The listing builds one solid part. Answer for the finished solid, in the listing's coordinates (mm). A direction names the side the tool comes from. Coordinates: 2 decimals unless noted, no trailing zeros. Write each loop counter-clockwise with the first axis right and the second up, starting at its lowest first coordinate (ties: lowest second). Pieces come first, ordered by that corner, then holes. Notation, with made-up numbers: M 10.25,3 L 30.25,3 A24 ccw 30.25,35 Z; hole C -1,58.5 d11. An arc over 180 degrees is marked long. Put each result on its own line as item: value. Start each with the question number.
```python
from build123d import *

# Parameters (mm, degrees)
SKETCH_1_R               = 2.5
EXTRUDE_1_DEPTH          = 86
HOLE_WIZARD_M3_1_D       = 2.5
HOLE_WIZARD_M3_1_DEPTH   = 6.748924226
HOLE_WIZARD_M3_1_TIP     = 0.751075774
HOLE_WIZARD_M3_2_D       = 2.5
HOLE_WIZARD_M3_2_DEPTH   = 6.748924226
HOLE_WIZARD_M3_2_TIP     = 0.751075774
CUT_EXTRUDE_2_DEPTH      = 5
CUT_EXTRUDE_2_DEPTH_BACK = 5
SKETCH_10_R              = 1.5
SKETCH_10_R_2            = 1.4


with BuildPart() as part:
    # Sketch 1 → Extrude 1 (new body)
    with BuildSketch(Plane(origin=(0, 0, 0), x_dir=(1, 0, 0), z_dir=(0, 1, 0))):
        with Locations(Location((0, 0, 0), (0, 0, 270))):
            Circle(SKETCH_1_R)
    extrude(amount=EXTRUDE_1_DEPTH)

    # Hole Wizard M3 _1
    with Locations(Plane(origin=(0, 0, 0), x_dir=(-1, 0, 0), z_dir=(0, -1, 0))):
        with Locations((0, 0)):
            Hole(HOLE_WIZARD_M3_1_D / 2, depth=HOLE_WIZARD_M3_1_DEPTH)
            with Locations((0, 0, -(HOLE_WIZARD_M3_1_DEPTH + HOLE_WIZARD_M3_1_TIP / 2))):  # 118° drill point
                Cone(0, HOLE_WIZARD_M3_1_D / 2, HOLE_WIZARD_M3_1_TIP, mode=Mode.SUBTRACT)

    # Hole Wizard M3 _2
    with Locations(Plane(origin=(0, 86, 0), x_dir=(1, 0, 0), z_dir=(0, 1, 0))):
        with Locations((0, 0)):
            Hole(HOLE_WIZARD_M3_2_D / 2, depth=HOLE_WIZARD_M3_2_DEPTH)
            with Locations((0, 0, -(HOLE_WIZARD_M3_2_DEPTH + HOLE_WIZARD_M3_2_TIP / 2))):  # 118° drill point
                Cone(0, HOLE_WIZARD_M3_2_D / 2, HOLE_WIZARD_M3_2_TIP, mode=Mode.SUBTRACT)

    # Sketch 10 → Cut-Extrude 2 (cut, two sides: drawn at the far end of the back side and taken through both)
    with BuildSketch(Plane(origin=(0, 0, 0), x_dir=(0, 0, -1), z_dir=(1, 0, 0)).offset(-CUT_EXTRUDE_2_DEPTH_BACK)):
        with Locations(Location((0, 68, 0), (0, 0, 180))):
            Circle(SKETCH_10_R)
        with Locations(Location((0, 9, 0), (0, 0, 180))):
            Circle(SKETCH_10_R_2)
    extrude(amount=CUT_EXTRUDE_2_DEPTH + CUT_EXTRUDE_2_DEPTH_BACK, mode=Mode.SUBTRACT)


solid = part.part
```
1) Determine the mould class of faces 1 (the face through (-0.04, 67.93, -1.5)), 2 (the face through (-0.05, 78.63, 0.21)), 3 (the face through (0.27, 82.58, 1.22)) for opening direction Y: +Y half, -Y half, draft (parallel to the pull), parting line (faces both ways), or undercut.
2) Straight lines are drawn through the part: probe 1 along Y at (x, z) = (2.2, 1); probe 2 along Y at (x, z) = (2.2, -0.2); probe 3 along X at (y, z) = (38.5, 2). For each, find the intervals that lie inside material, in ascending order.
3) A cutting plane is placed at A-A on y = 68. Write down the section's boundary in (x, z), then the cut area to 3 significant figures.
4) Given pin 1 Ø2 at (y, z) = (9, 0) entering from +X; pin 2 Ø2 at (x, z) = (0, 0) entering from -Y, each flat-ended and moving along its own axis, determine where each tip first touches the part or whether it passes through.
5) A cutting plane is placed at B-B on y = 44. Write down the section's boundary in (x, z), then the cut area to 3 significant figures.
6) For faces 4 (the face through (-2.44, 42.4, -0.54)), 5 (the face through (-0.27, 3.42, 1.22)), determine the directions among +Z, -Z, +X, -X, +Y, -Y from which every point of the face is accessible in a straight line to the end or side of a thin tool.
Answers follow:
1. face 1: undercut
1. face 2: +Y half
1. face 3: draft
2. probe 1: y = 0 to 8.02, 9.98 to 66.88, 69.12 to 86
2. probe 2: y = 0 to 7.61, 10.39 to 66.51, 69.49 to 86
2. probe 3: x = -1.5 to 1.5
3. outline: M -2,-1.5 A2.5 ccw 2,-1.5 Z; M -2,1.5 L 2,1.5 A2.5 ccw Z
3. area: 5.59 mm²
4. pin 1: passes through
4. pin 2: stops at y = 6.9
5. outline: C 0,0 d5
5. area: 19.6 mm²
6. face 4: +Y, -Y
6. face 5: -Y
